Build history of the part. All positions in model axes, mm. A direction names the side the tool comes from. Give positions to 0.01 mm unless a question says otherwise; leave off trailing zeros. Order: outer loops, then holes, each group sorted by start corner. A loop starts at its lowest first (then second) coordinate and runs counter-clockwise, first axis right, second up. Notation, with made-up numbers: (80.5, 55.5) - (119.5, 55.5) arc R24 ccw to (119.5, 87.5) - close; hole circle Ø11 at (58.5, 77.25). An arc over 180 degrees is marked (long way). Answer in a Markdown table with one row per item.
```python
from build123d import *

# Parameters (mm, degrees)
SKETCH1_W                                  = 135
SKETCH1_H                                  = 25
BOSS_EXTRUDE1_DEPTH                        = 8
SKETCH2_W                                  = 15
SKETCH2_H                                  = 10
BOSS_EXTRUDE2_DEPTH                        = 8
FILLET1_R                                  = 5
SKETCH3_R                                  = 2
CUT_EXTRUDE1_DEPTH                         = 10
CUT_EXTRUDE2_DEPTH                         = 4
MIRROR3_AT_THE_SECOND_PLANE_COPY_1_SKETC_W = 15
MIRROR3_AT_THE_SECOND_PLANE_COPY_1_SKETC_H = 10
MIRROR3_AT_THE_SECOND_PLANE_COPY_1_DEPTH   = 8
MIRROR3_AT_THE_SECOND_PLANE_COPY_2_SKETC_R = 2
MIRROR3_AT_THE_SECOND_PLANE_COPY_2_DEPTH   = 10
MIRROR3_AT_THE_SECOND_PLANE_COPY_3_DEPTH   = 4
FILLET2_R                                  = 5
SKETCH5_R                                  = 2
CUT_EXTRUDE3_DEPTH                         = 10
SKETCH6_W                                  = 135
SKETCH6_H                                  = 12
CUT_EXTRUDE4_DEPTH                         = 4


with BuildPart() as part:
    # Sketch1 → Boss-Extrude1 (new body)
    with BuildSketch(Plane(origin=(0, 0, 0), x_dir=(1, 0, 0), z_dir=(0, 1, 0))):
        with Locations((67.5, 12.5)):
            Rectangle(SKETCH1_W, SKETCH1_H)
    extrude(amount=BOSS_EXTRUDE1_DEPTH)

    # Sketch2 → Boss-Extrude2 (add)
    with BuildSketch(Plane(origin=(0, 8, 0), x_dir=(1, 0, 0), z_dir=(0, 1, 0))):
        with Locations((7.5, 30)):
            Rectangle(SKETCH2_W, SKETCH2_H)
    boss_extrude2 = extrude(amount=-BOSS_EXTRUDE2_DEPTH)

    # Fillet1
    fillet1_edges = [part.edges().sort_by_distance(p)[0] for p in [
        (0, 4, -35),
        (15, 4, -35),
    ]]
    fillet(fillet1_edges, radius=FILLET1_R)

    # Sketch3 → Cut-Extrude1 (cut)
    with BuildSketch(Plane(origin=(0, 8, 0), x_dir=(1, 0, 0), z_dir=(0, 1, 0))):
        with Locations(Location((7.5, 30, 0), (0, 0, 270))):
            Circle(SKETCH3_R)
    cut_extrude1 = extrude(amount=-CUT_EXTRUDE1_DEPTH, mode=Mode.SUBTRACT)

    # Sketch4 → Cut-Extrude2 (cut)
    with BuildSketch(Plane(origin=(0, 8, 0), x_dir=(1, 0, 0), z_dir=(0, 1, 0))):
        with BuildLine():
            Line((3, 30), (3, 34.582575695))
            Line((3, 34.582575695), (3.751281218, 37.139462948))
            Line((3.751281218, 37.139462948), (12, 36.532200332))
            Line((12, 36.532200332), (12, 30))
            ThreePointArc((12, 30), (7.5, 25.5), (3, 30))
        make_face()
    cut_extrude2 = extrude(amount=-CUT_EXTRUDE2_DEPTH, mode=Mode.SUBTRACT)

    # Mirror3: Boss-Extrude2, Cut-Extrude1, Cut-Extrude2 across plane
    add(boss_extrude2.mirror(Plane.XY.offset(-12.5)))
    add(cut_extrude1.mirror(Plane.XY.offset(-12.5)), mode=Mode.SUBTRACT)
    add(cut_extrude2.mirror(Plane.XY.offset(-12.5)), mode=Mode.SUBTRACT)

    # Mirror3 at the second plane: Boss-Extrude2, Cut-Extrude1, Cut-Extrude2 across plane
    add(boss_extrude2.mirror(Plane.ZY.offset(-67.5)))
    add(cut_extrude1.mirror(Plane.ZY.offset(-67.5)), mode=Mode.SUBTRACT)
    add(cut_extrude2.mirror(Plane.ZY.offset(-67.5)), mode=Mode.SUBTRACT)

    # Mirror3 at the second plane copy 1 sketc → Mirror3 at the second plane copy 1 (add)
    with BuildSketch(Plane(origin=(135, 8, -25), x_dir=(-1, 0, 0), z_dir=(0, 1, 0))):
        with Locations((7.5, 30)):
            Rectangle(MIRROR3_AT_THE_SECOND_PLANE_COPY_1_SKETC_W, MIRROR3_AT_THE_SECOND_PLANE_COPY_1_SKETC_H)
    extrude(amount=-MIRROR3_AT_THE_SECOND_PLANE_COPY_1_DEPTH)

    # Mirror3 at the second plane copy 2 sketc → Mirror3 at the second plane copy 2 (cut)
    with BuildSketch(Plane(origin=(135, 8, -25), x_dir=(-1, 0, 0), z_dir=(0, 1, 0))):
        with Locations(Location((7.5, 30, 0), (0, 0, 270))):
            Circle(MIRROR3_AT_THE_SECOND_PLANE_COPY_2_SKETC_R)
    extrude(amount=-MIRROR3_AT_THE_SECOND_PLANE_COPY_2_DEPTH, mode=Mode.SUBTRACT)

    # Mirror3 at the second plane copy 3 sketc → Mirror3 at the second plane copy 3 (cut)
    with BuildSketch(Plane(origin=(135, 8, -25), x_dir=(-1, 0, 0), z_dir=(0, 1, 0))):
        with BuildLine():
            Line((3, 30), (3, 34.582575695))
            Line((3, 34.582575695), (3.751281218, 37.139462948))
            Line((3.751281218, 37.139462948), (12, 36.532200332))
            Line((12, 36.532200332), (12, 30))
            ThreePointArc((12, 30), (7.5, 25.5), (3, 30))
        make_face()
    extrude(amount=-MIRROR3_AT_THE_SECOND_PLANE_COPY_3_DEPTH, mode=Mode.SUBTRACT)

    # Fillet2
    fillet2_edges = [part.edges().sort_by_distance(p)[0] for p in [
        (15, 4, -25),
        (120, 4, -35),
        (120, 4, -25),
        (135, 4, -35),
        (15, 4, 10),
        (15, 4, 0),
        (0, 4, 10),
        (135, 4, 10),
        (120, 4, 10),
        (120, 4, 0),
    ]]
    fillet(fillet2_edges, radius=FILLET2_R - 0.0001)  # a hair under: the kernel refuses the full size

    # Sketch5 → Cut-Extrude3 (cut)
    with BuildSketch(Plane(origin=(0, 8, 0), x_dir=(1, 0, 0), z_dir=(0, 1, 0))):
        with Locations(Location((10, 12.5, 0), (0, 0, 270))):
            Circle(SKETCH5_R)
        with Locations(Location((30, 12.5, 0), (0, 0, 270))):
            Circle(SKETCH5_R)
        with Locations(Location((50, 12.5, 0), (0, 0, 270))):
            Circle(SKETCH5_R)
        with Locations(Location((60, 12.5, 0), (0, 0, 270))):
            Circle(SKETCH5_R)
        with Locations(Location((80, 12.5, 0), (0, 0, 270))):
            Circle(SKETCH5_R)
        with Locations(Location((100, 12.5, 0), (0, 0, 270))):
            Circle(SKETCH5_R)
        with Locations(Location((110, 12.5, 0), (0, 0, 270))):
            Circle(SKETCH5_R)
        with Locations(Location((130, 12.5, 0), (0, 0, 270))):
            Circle(SKETCH5_R)
    extrude(amount=-CUT_EXTRUDE3_DEPTH, mode=Mode.SUBTRACT)

    # Sketch6 → Cut-Extrude4 (cut)
    with BuildSketch(Plane.XZ):
        with Locations((67.5, -12.5)):
            Rectangle(SKETCH6_W, SKETCH6_H)
    extrude(amount=-CUT_EXTRUDE4_DEPTH, mode=Mode.SUBTRACT)


solid = part.part
```
1. Two-plate mould, pull along X, no slides. Class faces 6 (the face through (11.352, 6.028, -13.974)), 7 (the face through (68, 0, -2)), 8 (the face through (0, 5, -13)): +X half, -X half, draft (parallel to the pull), parting line (faces both ways), or undercut.
Check result:
| item | result |
|---|---|
| face 6 | undercut |
| face 7 | draft |
| face 8 | -X half |
2. Which spindle directions (+Z, -Z, +X, -X, +Y, -Y) get a long thin tool onto all of the face, cutting with end or side? Do faces 1 (the face through (127.4, 6, -25.5)), 2 (the face through (122, 4, 9)), 3 (the face through (67, 2, -6.5)), 4 (the face through (61.983, 6.028, -12.76)), 5 (the face through (127.4, 6, 0.5)). Say none if no direction does.
Check result:
| item | result |
|---|---|
| face 1 | -Z, +Y |
| face 2 | +Z, +Y, -Y |
| face 3 | +X, -X, -Y |
| face 4 | +Y, -Y |
| face 5 | +Z, +Y |
3. Cut at B-B on x = 80. Write the cut outline in (y, z).
Check result:
| item | result |
|---|---|
| outline | (0, -25) - (8, -25) - (8, -14.5) - (4, -14.5) - (4, -18.5) - (0, -18.5) - close; (0, -6.5) - (4, -6.5) - (4, -10.5) - (8, -10.5) - (8, 0) - (0, 0) - close |
4. Probe line 1 (Z direction, x = 127.5, y = 1.25); line 2 (Z direction, x = 52, y = 2); line 3 (Z direction, x = 12, y = 1.25). List the from-to ranges inside material, lowest first.
Check result:
| item | result |
|---|---|
| line 1 | z = -35 to -32, -28 to -18.5, -6.5 to 3, 7 to 10 |
| line 2 | z = -25 to -18.5, -6.5 to 0 |
| line 3 | z = -34.58 to -18.5, -6.5 to 9.58 |
5. Drop flat-ended pins along their axis: P1, Ø2, axis at x = 94.5, y = 3.5, coming from the +Z side; P2, Ø4.5, axis at y = 5, z = -32.5, coming from the -X side; P3, Ø5, axis at x = 127.5, z = 5, coming from the +Y side; P4, Ø3, axis at x = 7.5, z = -30, coming from the -Y side. Give the stop position or say it passes through.
Check result:
| item | result |
|---|---|
| P1 | stops at z = 0 |
| P2 | stops at x = 0.01 |
| P3 | stops at y = 4 |
| P4 | passes through |
6. Cut at A-A on y = 2.75. Count the separate pieces of the cut face and the enclosed holes in it, and give its area (3 significant figures).
Check result:
| item | result |
|---|---|
| separate pieces | 2 |
| enclosed holes | 4 |
| area | 2,280 mm² |
